The listing builds one solid part. Answer for the finished solid, in the listing's coordinates (mm). A direction names the side the tool comes from. Coordinates: 2 decimals unless noted, no trailing zeros. Write each loop counter-clockwise with the first axis right and the second up, starting at its lowest first coordinate (ties: lowest second). Pieces come first, ordered by that corner, then holes.
(1) The part is cut by section B-B on z = -158.5. Determine the outline of the cut face in (x, y), plus the area to 3 significant figures.
(2) The part is cut by section A-A on x = 101.6. Give the number of separate pieces and of enclosed holes in the cut face, plus the area to 3 significant figures.
(3) For a pull along X with two mould halves and no side action, classify faces 3 (the flat face through (0, 3, -98)), 4 (the flat face through (77.383, 3.219, -119.806)), 5 (the cylindrical face through (118.135, 1.878, -87.44)) as +X half, -X half, draft (parallel to the pull), parting line (faces both ways), or undercut.
(4) Given P1, Ø6, axis at x = 98.5, z = -149.5, coming from the -Y side; P2, Ø3, axis at y = -3, z = -133, coming from the +X side; P3, Ø3, axis at x = 99, z = -99, coming from the -Y side, each flat-ended and moving along its own axis, determine where each tip first touches the part or whether it passes through.
(5) The part is cut by section C-C on y = -4. Determine the outline of the cut face in (x, z).
(6) Which of the six approach directions +Z, -Z, +X, -X, +Y, -Y give full straight-line access (tool end or side, diameter ignored) to faces 1 (the flat face through (81, 3.81, -111)), 2 (the flat face through (52.42, 3.219, -21.267))?
(7) The part is cut by section D-D on z = -81. Determine the outline of the cut face in (x, y), plus the area to 3 significant figures.
(8) Straight lines are drawn through the part: line 1 (Z direction, x = 192.5, y = 4.5); line 2 (X direction, y = 5, z = -121.5); line 3 (Z direction, x = 142, y = 1). For each, find the intervals that lie inside material, in ascending order.
from build123d import *

# Parameters (mm, degrees)
BOSS_EXTRUDE1_DEPTH     = 6.35
SKETCH3_R               = 2.286
CUT_EXTRUDE2_DEPTH      = 7.35
SKETCH4_R               = 2.286
CUT_EXTRUDE3_DEPTH      = 7.35
SKETCH5_W               = 184.404
SKETCH5_H               = 113.157
SKETCH5_R               = 2.286
BOSS_EXTRUDE2_DEPTH     = 6.35
FILLET1_R               = 6.35
BOSS_EXTRUDE3_DEPTH     = 6.35
SKETCH8_R               = 4.826
SKETCH8_R_2             = 2.286
BOSS_EXTRUDE4_DEPTH     = 6.35
SKETCH9_R               = 3.8354
CUT_EXTRUDE4_DEPTH      = 3.81
SKETCH11_R              = 2.286
CUT_EXTRUDE6_DEPTH      = 7.35
CUT_EXTRUDE6_DEPTH_BACK = 7.35
SKETCH12_R              = 4.7625
CUT_EXTRUDE7_DEPTH      = 6.35
SKETCH16_W              = 12.7
SKETCH16_H              = 12.7
BOSS_EXTRUDE6_DEPTH     = 5.08


with BuildPart() as part:
    # Sketch1 → Boss-Extrude1 (new body)
    with BuildSketch(Plane(origin=(0, 0, 0), x_dir=(1, 0, 0), z_dir=(0, 1, 0))):
        Polygon((0, 192.024), (6.35, 198.374), (196.85, 198.374), (203.2, 192.024), (203.2, 6.35), (196.85, 0), (6.35, 0), (0, 6.35), align=None)
    extrude(amount=BOSS_EXTRUDE1_DEPTH)

    # Sketch3 → Cut-Extrude2 (cut, through all)
    with BuildSketch(Plane(origin=(0, 6.35, 0), x_dir=(1, 0, 0), z_dir=(0, 1, 0))):
        with Locations((11.73734, 11.73734)):
            Circle(SKETCH3_R)
        with Locations((191.46266, 11.73734)):
            Circle(SKETCH3_R)
        with Locations((191.46266, 186.63666)):
            Circle(SKETCH3_R)
        with Locations((11.73734, 186.63666)):
            Circle(SKETCH3_R)
    extrude(amount=-CUT_EXTRUDE2_DEPTH, mode=Mode.SUBTRACT)

    # Sketch4 → Cut-Extrude3 (cut, through all)
    with BuildSketch(Plane(origin=(0, 6.35, 0), x_dir=(1, 0, 0), z_dir=(0, 1, 0))):
        with Locations((15.748, 149.4155)):
            Circle(SKETCH4_R)
        with Locations((187.452, 149.4155)):
            Circle(SKETCH4_R)
        with Locations((187.452, 48.9585)):
            Circle(SKETCH4_R)
        with Locations((15.748, 48.9585)):
            Circle(SKETCH4_R)
        Polygon((12.573, 137.260243879), (64.490719308, 189.177963187), (138.709280692, 189.177963187), (190.627, 137.260243879), (190.627, 61.113756121), (138.709280692, 9.196036813), (64.490719308, 9.196036813), (12.573, 61.113756121), align=None)
    extrude(amount=-CUT_EXTRUDE3_DEPTH, mode=Mode.SUBTRACT)

    # Sketch5 → Boss-Extrude2 (add)
    with BuildSketch(Plane(origin=(0, 6.35, 0), x_dir=(1, 0, 0), z_dir=(0, 1, 0))):
        with Locations((101.6, 99.187)):
            Rectangle(SKETCH5_W, SKETCH5_H)
        with Locations((187.452, 48.9585)):
            Circle(SKETCH5_R, mode=Mode.SUBTRACT)
        with Locations((187.452, 149.4155)):
            Circle(SKETCH5_R, mode=Mode.SUBTRACT)
        with Locations((15.748, 149.4155)):
            Circle(SKETCH5_R, mode=Mode.SUBTRACT)
        with Locations((15.748, 48.9585)):
            Circle(SKETCH5_R, mode=Mode.SUBTRACT)
        with BuildLine():
            Line((143.313899503, 143.0655), (59.886100497, 143.0655))
            ThreePointArc((59.886100497, 143.0655), (53.736909414, 138.299781862), (56.817737694, 131.156035124))
            Line((56.817737694, 131.156035124), (98.531637197, 108.133427651))
            ThreePointArc((98.531637197, 108.133427651), (101.6, 107.342892527), (104.668362803, 108.133427651))
            Line((104.668362803, 108.133427651), (146.382262306, 131.156035124))
            ThreePointArc((146.382262306, 131.156035124), (149.463090586, 138.299781862), (143.313899503, 143.0655))
        make_face(mode=Mode.SUBTRACT)
        with BuildLine():
            Line((22.098, 125.054934949), (22.098, 73.319065051))
            ThreePointArc((22.098, 73.319065051), (25.220121734, 67.850673889), (31.516362803, 67.759600175))
            Line((31.516362803, 67.759600175), (78.385616864, 93.627535124))
            ThreePointArc((78.385616864, 93.627535124), (81.667254061, 99.187), (78.385616864, 104.746464876))
            Line((78.385616864, 104.746464876), (31.516362803, 130.614399825))
            ThreePointArc((31.516362803, 130.614399825), (25.220121734, 130.523326111), (22.098, 125.054934949))
        make_face(mode=Mode.SUBTRACT)
        with BuildLine():
            Line((59.886100497, 55.3085), (143.313899503, 55.3085))
            ThreePointArc((143.313899503, 55.3085), (149.463090586, 60.074218138), (146.382262306, 67.217964876))
            Line((146.382262306, 67.217964876), (104.668362803, 90.240572349))
            ThreePointArc((104.668362803, 90.240572349), (101.6, 91.031107473), (98.531637197, 90.240572349))
            Line((98.531637197, 90.240572349), (56.817737694, 67.217964876))
            ThreePointArc((56.817737694, 67.217964876), (53.736909414, 60.074218138), (59.886100497, 55.3085))
        make_face(mode=Mode.SUBTRACT)
        with BuildLine():
            Line((181.102, 73.319065051), (181.102, 125.054934949))
            ThreePointArc((181.102, 125.054934949), (177.979878266, 130.523326111), (171.683637197, 130.614399825))
            Line((171.683637197, 130.614399825), (124.814383136, 104.746464876))
            ThreePointArc((124.814383136, 104.746464876), (121.532745939, 99.187), (124.814383136, 93.627535124))
            Line((124.814383136, 93.627535124), (171.683637197, 67.759600175))
            ThreePointArc((171.683637197, 67.759600175), (177.979878266, 67.850673889), (181.102, 73.319065051))
        make_face(mode=Mode.SUBTRACT)
    extrude(amount=-BOSS_EXTRUDE2_DEPTH)

    # Fillet1
    fillet1_edges = [part.edges().sort_by_distance(p)[0] for p in [
        (64.490719308, 3.175, -189.177963187),
        (138.709280692, 3.175, -189.177963187),
        (138.709280692, 3.175, -9.196036813),
        (64.490719308, 3.175, -9.196036813),
        (31.078256121, 3.175, -42.6085),
        (172.121743879, 3.175, -155.7655),
        (31.078256121, 3.175, -155.7655),
        (172.121743879, 3.175, -42.6085),
    ]]
    fillet(fillet1_edges, radius=FILLET1_R)

    # Sketch6 → Boss-Extrude3 (add)
    with BuildSketch(Plane(origin=(0, 6.35, 0), x_dir=(1, 0, 0), z_dir=(0, 1, 0))):
        with BuildLine():
            Line((87.252770852, 9.196036813), (115.947229148, 9.196036813))
            ThreePointArc((115.947229148, 9.196036813), (109.135280152, 12.063486522), (106.424731926, 18.939375212))
            ThreePointArc((106.424731926, 18.939375212), (101.6, 23.876), (96.775268074, 18.939375212))
            ThreePointArc((96.775268074, 18.939375212), (94.064719848, 12.063486522), (87.252770852, 9.196036813))
        make_face()
    extrude(amount=-BOSS_EXTRUDE3_DEPTH)

    # Sketch8 → Boss-Extrude4 (add)
    with BuildSketch(Plane(origin=(0, 0, 0), x_dir=(1, 0, 0), z_dir=(0, 1, 0))):
        with Locations((101.6, 19.05)):
            Circle(SKETCH8_R)
        with Locations((101.6, 19.05)):
            Circle(SKETCH8_R_2, mode=Mode.SUBTRACT)
    extrude(amount=-BOSS_EXTRUDE4_DEPTH)

    # Sketch9 → Cut-Extrude4 (cut)
    with BuildSketch(Plane(origin=(0, 0, 0), x_dir=(1, 0, 0), z_dir=(0, 1, 0))):
        with Locations((81.233070117, 111.102859125)):
            Circle(SKETCH9_R)
        with Locations((121.966929883, 111.102859125)):
            Circle(SKETCH9_R)
        with Locations((121.966929883, 87.271140875)):
            Circle(SKETCH9_R)
        with Locations((81.233070117, 87.271140875)):
            Circle(SKETCH9_R)
    extrude(amount=CUT_EXTRUDE4_DEPTH, mode=Mode.SUBTRACT)

    # Sketch11 → Cut-Extrude6 (cut, two sides)
    with BuildSketch(Plane.XZ) as cut_extrude6_sk:
        with Locations((31.75, -12.7)):
            Circle(SKETCH11_R)
        with Locations((171.45, -12.7)):
            Circle(SKETCH11_R)
        with Locations((171.45, -185.674)):
            Circle(SKETCH11_R)
        with Locations((31.75, -185.674)):
            Circle(SKETCH11_R)
    extrude(amount=CUT_EXTRUDE6_DEPTH, mode=Mode.SUBTRACT)
    extrude(cut_extrude6_sk.sketch, amount=-CUT_EXTRUDE6_DEPTH_BACK, mode=Mode.SUBTRACT)

    # Sketch12 → Cut-Extrude7 (cut)
    with BuildSketch(Plane(origin=(0, 6.35, 0), x_dir=(1, 0, 0), z_dir=(0, 1, 0))):
        with Locations((100.413067708, 99.782171875)):
            Circle(SKETCH12_R)
    extrude(amount=-CUT_EXTRUDE7_DEPTH, mode=Mode.SUBTRACT)

    # Sketch16 → Boss-Extrude6 (add)
    with BuildSketch(Plane(origin=(0, 6.35, 0), x_dir=(1, 0, 0), z_dir=(0, 1, 0))):
        with Locations((100.413067708, 99.782171875)):
            Rectangle(SKETCH16_W, SKETCH16_H)
    extrude(amount=-BOSS_EXTRUDE6_DEPTH)


solid = part.part
Model answer:
1. outline: (0, 0) - (41.19, 0) - (41.19, 6.35) - (0, 6.35) - close; (162.01, 0) - (203.2, 0) - (203.2, 6.35) - (162.01, 6.35) - close
1. area: 523 mm2
2. separate pieces: 5
2. enclosed holes: 0
2. area: 495 mm2
3. face 3: -X half
3. face 4: undercut
3. face 5: undercut
4. P1: stops at y = 0
4. P2: passes through
4. P3: stops at y = 1.27
5. outline: circle Ø9.65 at (101.6, -19.05); hole circle Ø4.57 at (101.6, -19.05)
6. face 1: -Y
6. face 2: +Y, -Y
7. outline: (0, 0) - (22.1, 0) - (22.1, 6.35) - (0, 6.35) - close; (55.51, 0) - (81.79, 0) - (81.79, 6.35) - (55.51, 6.35) - close; (121.41, 0) - (147.69, 0) - (147.69, 6.35) - (121.41, 6.35) - close; (181.1, 0) - (203.2, 0) - (203.2, 6.35) - (181.1, 6.35) - close
7. area: 614 mm2
8. line 1: z = -198.37 to -188.67, -184.6 to -13.77, -9.7 to 0
8. line 2: x = 0 to 22.1, 48.03 to 74.31, 128.89 to 155.17, 181.1 to 203.2
8. line 3: z = -198.37 to -185.89, -155.77 to -143.07, -128.74 to -114.23, -84.14 to -69.64, -55.31 to -42.61, -12.49 to 0
